```python
from build123d import *

# Parameters (mm, degrees)
F0_W     = 25
F0_H     = 40
F2_ANGLE = 90
F1_W     = 15
F1_H     = 30
F3_ANGLE = 90
F4_DEPTH = 10
F5_DEPTH = 10


with BuildPart() as f2:
    # F0 (on Top) → F2 (revolve)
    with BuildSketch(Plane.XY):
        Rectangle(F0_W, F0_H)
    revolve(axis=Axis((-1.096226, -51.309453, 0), (1, 0, 0)), revolution_arc=F2_ANGLE)

    # F1 (on Top) → F3 (revolve, cut)
    with BuildSketch(Plane.XY):
        Rectangle(F1_W, F1_H)
    revolve(axis=Axis((-1.096226, -51.309453, 0), (1, 0, 0)), revolution_arc=F3_ANGLE, mode=Mode.SUBTRACT)

    # F0 (on Top) → F4 (join)
    with BuildSketch(Plane.XY):
        Rectangle(F0_W, F0_H)
    extrude(amount=-F4_DEPTH)

    # F1 (on Top) → F5 (cut)
    with BuildSketch(Plane.XY):
        Rectangle(F1_W, F1_H)
    extrude(amount=-F5_DEPTH, mode=Mode.SUBTRACT)


solid = f2.part
```
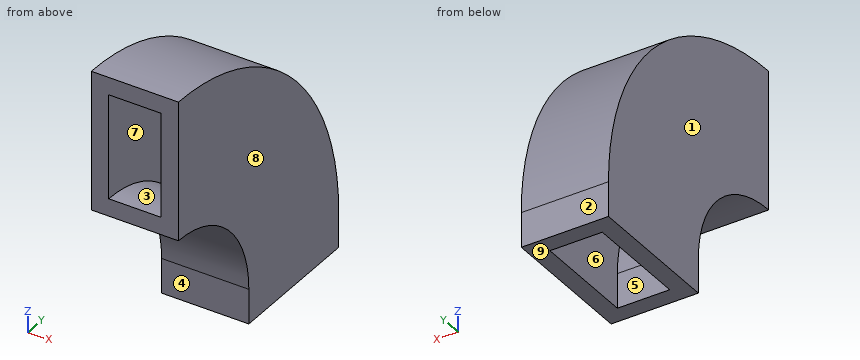
The listing builds one solid part. Answer for the finished solid, in the listing's coordinates (mm). Face numbers are marked on the shaded views. A direction names the side the tool comes from. Give positions to 0.01 mm unless a question says otherwise; leave off trailing zeros. Write each loop counter-clockwise with the first axis right and the second up, starting at its lowest first coordinate (ties: lowest second). Pieces come first, ordered by that corner, then holes. Notation, with made-up numbers: (52.25, 86) -> (64.25, 86) arc R27 cw to (64.25, 108) -> close; hole circle Ø6 at (-24, 17). An arc over 180 degrees is marked (long way). Use one line per item in the form item = value.
1) Section C-C on y = -46 is taken. Write down the section's boundary in (x, z), plus the area to 3 significant figures.
Result:
outline = (-12.5, 30.86) -> (12.5, 30.86) -> (12.5, 71.11) -> (-12.5, 71.11) -> close; hole (-7.5, 35.92) -> (7.5, 35.92) -> (7.5, 66.1) -> (-7.5, 66.1) -> close
area = 554 mm²
2) Section A-A on x = -5.25 is taken. Write down the section's boundary in (y, z), plus the area to 3 significant figures.
Result:
outline = (-51.31, 31.31) arc R31.31 cw to (-20, 0) -> (-20, -10) -> (-15, -10) -> (-15, 0) arc R36.31 ccw to (-51.31, 36.31) -> close; (-51.31, 66.31) arc R66.31 cw to (15, 0) -> (15, -10) -> (20, -10) -> (20, 0) arc R71.31 ccw to (-51.31, 71.31) -> close
area = 906 mm²
3) Each of these flat-tipped pins is pushed along its axis until it touches: P1, Ø5, axis at x = 2, z = -3.5, coming from the -Y side; P2, Ø5, axis at x = -7, z = 7.5, coming from the -Y side; P3, Ø1.5, axis at x = -9.5, y = 0, coming from the +Z side. Where does it stop, or does it pass through?
Result:
P1 = -20
P2 = -21.64
P3 = 50.29
4) Straight lines are drawn through the part: probe 1 along X at (y, z) = (-29, 32.5); probe 2 along Z at (x, y) = (-3.75, -29); probe 3 along Y at (x, z) = (0, 9.5). For each, find the intervals that lie inside material, in ascending order.
Result:
probe_1 = -12.5 to -7.5, 7.5 to 12.5
probe_2 = 21.97 to 28.65, 62.44 to 67.73
probe_3 = -21.48 to -16.26, 14.32 to 19.36
5) A tool of negligible diameter and unlimited length cuts with its end or side. For the marked faces 1, 2, 3, 4 and 5, from which of +Z, -Z, +X, -X, +Y, -Y can it reach the whole face along a straight path? Write none if from no direction.
Result:
face_1 = +Z, -Z, -X, +Y, -Y
face_2 = +Z, -Z, +X, -X, +Y
face_3 = none
face_4 = -Z, +X, -X, -Y
face_5 = -Z
6) Section D-D on z = 50 is taken. Write down the section's boundary in (x, y).
Result:
outline = (-12.5, -51.31) -> (-7.5, -51.31) -> (-7.5, -7.76) -> (7.5, -7.76) -> (7.5, -51.31) -> (12.5, -51.31) -> (12.5, -0.47) -> (-12.5, -0.47) -> close
7) Section B-B on z = -5 is taken. Write down the section's boundary in (x, y), plus the area to 3 significant figures.
Result:
outline = (-12.5, -20) -> (12.5, -20) -> (12.5, 20) -> (-12.5, 20) -> close; hole (-7.5, -15) -> (7.5, -15) -> (7.5, 15) -> (-7.5, 15) -> close
area = 550 mm²
8) For a pull along X with two mould halves and no side action, classify the marked faces 6, 7, 8 and 9 as +X half, -X half, draft (parallel to the pull), parting line (faces both ways), or undercut.
Result:
face_6 = undercut
face_7 = undercut
face_8 = +X half
face_9 = draft
